Part model, mm, in its own coordinate system. A direction names the side the tool comes from. Coordinates: 2 decimals unless noted, no trailing zeros. Loops run counter-clockwise (first coordinate to the right, second up) from the corner with the lowest first, then second, coordinate; pieces in that order, holes last. Notation, with made-up numbers: M -11.75,34.5 L 13.25,34.5 A17 ccw 13.25,42.5 Z; hole C -27.5,65 d10. An arc over 180 degrees is marked long. Answer as a JSON object with one key per item and string values. Group by question number.
1. Drop flat-ended pins along their axis: pin 1 Ø0.8 at (y, z) = (0.5, 3.5) entering from -X; pin 2 Ø1.5 at (x, y) = (11.5, 16.5) entering from -Z; pin 3 Ø2.5 at (x, z) = (9, 5) entering from -Y. Give the stop position or say it passes through.
2. Saw through at B-B on x = 7.72. Write the cut outline in (y, z), then the cut area to 3 significant figures.
3. Saw through at A-A on z = 3.5. Write the cut outline in (x, y), then the cut area to 3 significant figures.
4. Drill centre lines: L1, parallel to Z at x = 5.25, y = 6.5; L2, parallel to Y at x = 6.5, z = 2.25; L3, parallel to X at y = 6.5, z = 2.5. Where is each one in solid material? Low to high.
5. Saw through at D-D on x = 6. Write the cut outline in (y, z), then the cut area to 3 significant figures.
6. Saw through at C-C on z = 0.75. Write the cut outline in (x, y).
7. 3-axis set-ups, long thin cutter, end or side, ignore diameter. For faces 5 (the face through (14.14, 6.25, 7.86)), 6 (the face through (5.654, 15.512, 2.683)), 7 (the face through (1.88, 5.47, 4.04)): which of +Z, -Z, +X, -X, +Y, -Y reach the whole face in a straight line?
8. Mould opens along Y. For faces 1 (the face through (1.68, 6.97, 3.23)), 2 (the face through (8, 0, 7)), 3 (the face through (1.22, 6.08, 7.85)), 4 (the face through (13.243, 9.677, 2.261)) say: released by +Y, released by -Y, zero draft, split by the parting line, or undercut.
from build123d import *

# Parameters (mm, degrees)
BOSS_EXTRUDE1_DEPTH = 8
CUT_EXTRUDE3_START  = -1.5
CUT_EXTRUDE3_DEPTH  = 5
SKETCH2_R           = 1.96
CUT_EXTRUDE1_DEPTH  = 0.9
SKETCH3_R           = 2
CUT_EXTRUDE2_DEPTH  = 0.9
FILLET1_R           = 0.5
SKETCH4_R           = 2.45
BOSS_EXTRUDE2_DEPTH = 5.5


with BuildPart() as part:
    # Sketch1 → Boss-Extrude1 (new body)
    with BuildSketch(Plane.XY):
        Polygon((0, 0), (15.4, 0), (13.143014647, 12.8), (2.256985353, 12.8), align=None)
    extrude(amount=BOSS_EXTRUDE1_DEPTH)

    # Sketch5 → Cut-Extrude3 (cut)
    with BuildSketch(Plane.XY.offset(8).offset(CUT_EXTRUDE3_START)):
        Polygon((1.178374422, 0), (1.178374422, 1.5), (3.012175021, 11.9), (12.387824979, 11.9), (14.221625578, 1.5), (14.221625578, 0), align=None)
    extrude(amount=-CUT_EXTRUDE3_DEPTH, mode=Mode.SUBTRACT)

    # Sketch2 → Cut-Extrude1 (cut)
    with BuildSketch(Plane(origin=(14.93563318, 2.633555104, 0), x_dir=(0, 0, -1), z_dir=(0.9848077530122086, 0.17364817766692736, 0))):
        with Locations(Location((-4, 6.325818064, 0), (0, 0, 90))):
            Circle(SKETCH2_R)
    extrude(amount=-CUT_EXTRUDE1_DEPTH, mode=Mode.SUBTRACT)

    # Sketch3 → Cut-Extrude2 (cut)
    with BuildSketch(Plane(origin=(0, 0, 0), x_dir=(0, 0, 1), z_dir=(-0.9848077530122087, 0.17364817766692736, 0))):
        with Locations(Location((4, 9, 0), (0, 0, 270))):
            Circle(SKETCH3_R)
    extrude(amount=-CUT_EXTRUDE2_DEPTH, mode=Mode.SUBTRACT)

    # Fillet1
    fillet1_edges = [part.edges().sort_by_distance(p)[0] for p in [
        (14.271507323, 6.4, 8),
        (7.7, 12.8, 8),
        (1.128492677, 6.4, 8),
        (7.7, 12.8, 0),
        (14.271507323, 6.4, 0),
        (1.128492677, 6.4, 0),
        (2.256985353, 12.8, 4),
        (13.143014647, 12.8, 4),
    ]]
    fillet(fillet1_edges, radius=FILLET1_R)

    # Sketch4 → Boss-Extrude2 (add)
    with BuildSketch(Plane(origin=(0, 12.8, 0), x_dir=(1, 0, 0), z_dir=(0, 1, 0))):
        with Locations(Location((7.72, -4, 0), (0, 0, 90))):
            Circle(SKETCH4_R)
    extrude(amount=BOSS_EXTRUDE2_DEPTH)


solid = part.part
Outcome:
{
 "1": {"pin 1": "stops at x = 0.02", "pin 2": "passes through", "pin 3": "stops at y = 11.9"},
 "2": {"outline": "M 0,0 L 12.3,0 A0.5 ccw 12.8,0.5 L 12.8,1.55 L 18.3,1.55 L 18.3,6.45 L 12.8,6.45 L 12.8,7.5 A0.5 ccw 12.3,8 L 0,8 L 0,6.5 L 11.9,6.5 L 11.9,1.5 L 0,1.5 Z", "area": "69.7 mm²"},
 "3": {"outline": "M 0,0 L 1.18,0 L 1.18,1.5 L 2.11,6.8 L 1.23,6.96 Z; M 1.9,10.77 L 2.79,10.61 L 3.01,11.9 L 12.39,11.9 L 12.62,10.57 L 13.51,10.73 L 13.22,12.39 A0.5 ccw 12.72,12.8 L 10.12,12.8 L 10.12,18.3 L 5.32,18.3 L 5.32,12.8 L 2.68,12.8 A0.5 ccw 2.18,12.39 Z; M 13.28,6.84 L 14.22,1.5 L 14.22,0 L 15.4,0 L 14.17,7 Z", "area": "51.5 mm²"},
 "4": {"L1": "z = 0 to 1.5, 6.5 to 8", "L2": "y = 11.9 to 18.3", "L3": "x = 1.15 to 2.06, 13.34 to 14.25"},
 "5": {"outline": "M 0,0 L 12.3,0 A0.5 ccw 12.8,0.5 L 12.8,2.26 L 18.3,2.26 L 18.3,5.74 L 12.8,5.74 L 12.8,7.5 A0.5 ccw 12.3,8 L 0,8 L 0,6.5 L 11.9,6.5 L 11.9,1.5 L 0,1.5 Z", "area": "62.0 mm²"},
 "6": {"outline": "M 0,0 L 15.4,0 L 13.22,12.39 A0.5 ccw 12.72,12.8 L 2.68,12.8 A0.5 ccw 2.18,12.39 Z"},
 "7": {"face 5": "+Z, +X, +Y", "face 6": "+Y", "face 7": "-Y"},
 "8": {"face 1": "undercut", "face 2": "released by -Y", "face 3": "released by +Y", "face 4": "undercut"}
}
